from build123d import *

# Parameters (mm, degrees)
ESTRUSIONE_ESTRUSIONE1_DEPTH = 6.5
TAGLIO_ESTRUSIONE2_DEPTH     = 2.5
SCHIZZO2_R                   = 1.25
TAGLIO_ESTRUSIONE3_DEPTH     = 7.5
SCHIZZO4_W                   = 27
SCHIZZO4_H                   = 12.3
TAGLIO_ESTRUSIONE4_DEPTH     = 1.8
SCHIZZO6_R                   = 1.25
TAGLIO_ESTRUSIONE5_DEPTH     = 76


with BuildPart() as part:
    # Schizzo1 → Estrusione-Estrusione1 (new body)
    with BuildSketch(Plane.XY):
        Polygon((0, 0), (75, 0), (75, 33), (71.25, 33), (70, 11.85394892), (55, 11.85394892), (55, 15.118104456), (20, 15.118104456), (20, 11.85394892), (5, 11.85394892), (3.75, 33), (0, 33), align=None)
    extrude(amount=ESTRUSIONE_ESTRUSIONE1_DEPTH)

    # Schizzo3 → Taglio-Estrusione2 (cut)
    with BuildSketch(Plane(origin=(0, 0, 0), x_dir=(-1, 0, 0), z_dir=(0, 0, -1))):
        Polygon((-44.599573519, 9.5), (-46.18728676, 12.25), (-49.36271324, 12.25), (-50.950426481, 9.5), (-49.36271324, 6.75), (-46.18728676, 6.75), align=None)
        Polygon((-24.049573519, 9.5), (-25.63728676, 12.25), (-28.81271324, 12.25), (-30.400426481, 9.5), (-28.81271324, 6.75), (-25.63728676, 6.75), align=None)
    extrude(amount=-TAGLIO_ESTRUSIONE2_DEPTH, mode=Mode.SUBTRACT)

    # Schizzo2 → Taglio-Estrusione3 (cut, through all)
    with BuildSketch(Plane.XY.offset(6.5)):
        with Locations((27.225, 9.5)):
            Circle(SCHIZZO2_R)
        with Locations((47.775, 9.5)):
            Circle(SCHIZZO2_R)
    extrude(amount=-TAGLIO_ESTRUSIONE3_DEPTH, mode=Mode.SUBTRACT)

    # Schizzo4 → Taglio-Estrusione4 (cut)
    with BuildSketch(Plane.XY.offset(6.5)):
        with Locations((37.496683744, 6.15)):
            Rectangle(SCHIZZO4_W, SCHIZZO4_H)
    extrude(amount=-TAGLIO_ESTRUSIONE4_DEPTH, mode=Mode.SUBTRACT)

    # Schizzo6 → Taglio-Estrusione5 (cut, through all)
    with BuildSketch(Plane.ZY):
        with Locations((3.25, 25)):
            Circle(SCHIZZO6_R)
    extrude(amount=-TAGLIO_ESTRUSIONE5_DEPTH, mode=Mode.SUBTRACT)


solid = part.part
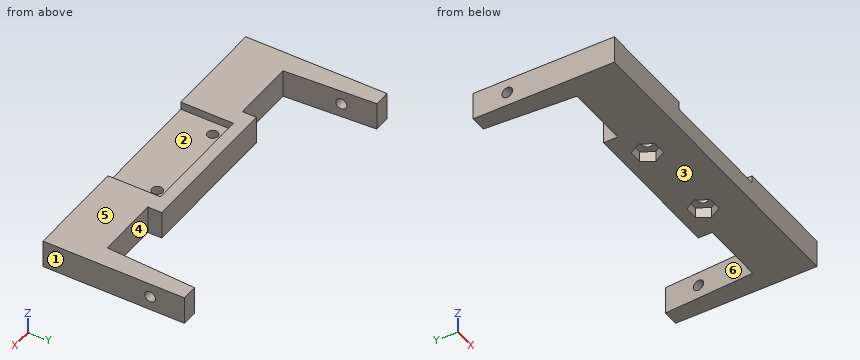
Read the model definition and answer for the solid it produces. Units are mm, in the model's axes. Face numbers are marked on the shaded views. A direction names the side the tool comes from. Round coordinates to 2 decimals unless told otherwise and drop trailing zeros. Loops run counter-clockwise (first coordinate to the right, second up) from the corner with the lowest first, then second, coordinate; pieces in that order, holes last. Notation, with made-up numbers: (-1.75, 63.5) - (51.25, 63.5) arc R20 ccw to (51.25, 72.5) - close; hole circle Ø8 at (-31, -37). An arc over 180 degrees is marked (long way). One line per question, with ' | ' between items. Start each with the question number.
Q1. Flat-ended cylindrical pins translate along their axes: pin 1 (3.5 mm diameter, centred on x = 39.5, y = 8, fed in from +Z); pin 2 (3 mm diameter, centred on x = 27, y = 10.5, fed in from -Z); pin 3 (0.8 mm diameter, centred on x = 47.5, z = 1.5, fed in from +Y). Find the tip coordinate at first contact, or state that the pin passes through.
Q2. Section B-B on y = 25 is taken. Give the vertices of the cut face in (x, z), plus the area to 3 significant figures.
Q3. Section D-D on y = 18 is taken. Give the vertices of the cut face in (x, z), plus the area to 3 significant figures.
Q4. For the marked faces 5 and 6, determine the directions among +Z, -Z, +X, -X, +Y, -Y from which every point of the face is accessible in a straight line to the end or side of a thin tool.
Q5. Find the intervals of material crossed by L1, parallel to X at y = 8.5, z = 4.25 (3 decimals); L2, parallel to Z at x = 72.65, y = 25; L3, parallel to Y at x = 72.15, z = 3.25, in increasing order.
Q6. Section C-C on z = 3.25 is taken. Give the vertices of the cut face in (x, y) (3 decimals), plus the area to 3 significant figures.
Q7. For a pull along X with two mould halves and no side action, classify the marked faces 1, 2, 3 and 4 as +X half, -X half, draft (parallel to the pull), parting line (faces both ways), or undercut.
Q8. Section A-A on x = 27 is taken. Give the vertices of the cut face in (y, z), plus the area to 3 significant figures.
Established:
1) pin 1: z = 4.7 | pin 2: z = 2.5 | pin 3: y = 15.12
2) outline: (0, 0) - (4.22, 0) - (4.22, 2) - (0, 2) - close; (0, 4.5) - (4.22, 4.5) - (4.22, 6.5) - (0, 6.5) - close; (70.78, 0) - (75, 0) - (75, 2) - (70.78, 2) - close; (70.78, 4.5) - (75, 4.5) - (75, 6.5) - (70.78, 6.5) - close | area: 33.8 mm²
3) outline: (0, 0) - (4.64, 0) - (4.64, 6.5) - (0, 6.5) - close; (70.36, 0) - (75, 0) - (75, 6.5) - (70.36, 6.5) - close | area: 60.3 mm²
4) face 5: +Z, +X, -X, +Y, -Y | face 6: +Z, -Z, +Y
5) L1: 0 to 26.475, 27.975 to 47.025, 48.525 to 75 | L2: 0 to 2, 4.5 to 6.5 | L3: 0 to 23.75, 26.25 to 33
6) outline: (0, 0) - (75, 0) - (75, 23.75) - (70.703, 23.75) - (70, 11.854) - (55, 11.854) - (55, 15.118) - (20, 15.118) - (20, 11.854) - (5, 11.854) - (4.297, 23.75) - (0, 23.75) - close; (0, 26.25) - (4.149, 26.25) - (3.75, 33) - (0, 33) - close; (70.851, 26.25) - (75, 26.25) - (75, 33) - (71.25, 33) - close; hole circle Ø2.5 at (27.225, 9.5); hole circle Ø2.5 at (47.775, 9.5) | area: 1,160 mm²
7) face 1: +X half | face 2: undercut | face 3: draft | face 4: undercut
8) outline: (0, 0) - (6.75, 0) - (6.75, 2.5) - (8.27, 2.5) - (8.27, 4.7) - (0, 4.7) - close; (10.73, 2.5) - (12.25, 2.5) - (12.25, 0) - (15.12, 0) - (15.12, 6.5) - (12.3, 6.5) - (12.3, 4.7) - (10.73, 4.7) - close | area: 57.0 mm²
